The model under review builds one solid part; all positions refer to its coordinate system, in mm. Face numbers are marked on the shaded views. A direction names the side the tool comes from. Give positions to 0.01 mm unless a question says otherwise; leave off trailing zeros. Loops run counter-clockwise (first coordinate to the right, second up) from the corner with the lowest first, then second, coordinate; pieces in that order, holes last. Notation, with made-up numbers: (1.5, 76) - (18.5, 76) arc R34 cw to (18.5, 106) - close; hole circle Ø3 at (65.5, 54). An arc over 180 degrees is marked (long way). Return JSON: item names as keys, results as strings. Group by question number.
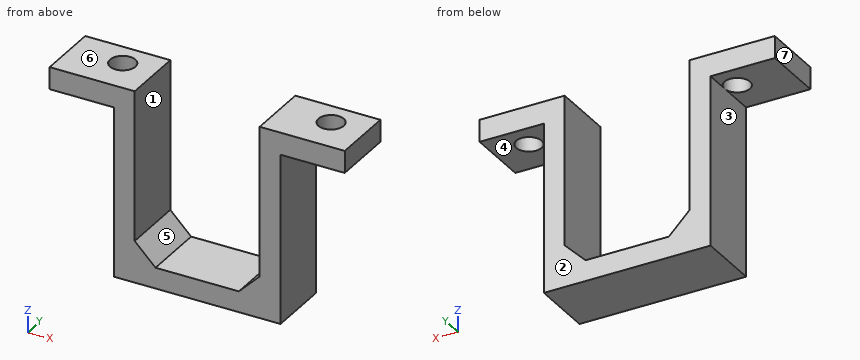
from build123d import *

# Parameters (mm, degrees)
BOSS_EXTRUDE1_DEPTH = 15
SKETCH3_R           = 3.05
CUT_EXTRUDE1_DEPTH  = 15


with BuildPart() as part:
    # Sketch2 → Boss-Extrude1 (new body)
    with BuildSketch(Plane(origin=(0, 0, 0), x_dir=(1, 0, 0), z_dir=(0, 1, 0))):
        Polygon((-13.5, 0), (6.5, 0), (11.5, -5), (11.5, -41), (31.917309801, -41), (31.917309801, -35.69895288), (16.5, -35.69895288), (16.5, 5), (-23.5, 5), (-23.5, -35.69895288), (-38.917309801, -35.69895288), (-38.917309801, -41), (-18.5, -41), (-18.5, -5), align=None)
    extrude(amount=BOSS_EXTRUDE1_DEPTH)

    # Sketch3 → Cut-Extrude1 (cut)
    with BuildSketch(Plane(origin=(0, 0, 35.69895288), x_dir=(-1, 0, 0), z_dir=(0, 0, -1))):
        with Locations((26.5, 9)):
            Circle(SKETCH3_R)
        with Locations((-23.5, 9)):
            Circle(SKETCH3_R)
    extrude(amount=-CUT_EXTRUDE1_DEPTH, mode=Mode.SUBTRACT)


solid = part.part
Item 1: Take a section at B-B (z = 29). State the section outline as (x, y) points, then the cut area to 3 significant figures.
Item 2: Take a section at D-D (x = 23.5). State the section outline as (y, z) points, then the cut area to 3 significant figures.
Item 3: Take a section at A-A (z = 37). State the section outline as (x, y) points.
Item 4: For L1, parallel to X at y = 9, z = 20.5; L2, parallel to X at y = 8, z = 37; L3, parallel to Z at x = -31.5, y = 12.75, list the stretches that pass through material, from the lowest coordinate up. Write a range as from..to.
Item 5: Take a section at C-C (y = 10.5). State the section outline as (x, z) points.
Item 6: Tool access review of the marked faces 1, 2, 3 and 4: name each direction out of +Z, -Z, +X, -X, +Y, -Y from which nothing blocks a thin tool from reaching the whole face with its end or side.
Item 7: For P1, Ø4.5, axis at y = 7.5, z = 30.5, coming from the +X side; P2, Ø3, axis at y = 6, z = 6, coming from the -X side; P3, Ø7, axis at x = 23.5, y = 9, coming from the -Z side, all flat-tipped, find the tip position at first contact; note any pin that passes through.
Item 8: Mouldability with a two-part tool opening along X and no side actions: class the marked faces 5, 6 and 7 as +X half, -X half, draft (parallel to the pull), parting line (faces both ways), or undercut.
Check sheet entries:
{
 "1": {"outline": "(-23.5, 0) - (-18.5, 0) - (-18.5, 15) - (-23.5, 15) - close; (11.5, 0) - (16.5, 0) - (16.5, 15) - (11.5, 15) - close", "area": "150 mm^2"},
 "2": {"outline": "(0, 35.7) - (5.95, 35.7) - (5.95, 41) - (0, 41) - close; (12.05, 35.7) - (15, 35.7) - (15, 41) - (12.05, 41) - close", "area": "47.2 mm^2"},
 "3": {"outline": "(-38.92, 0) - (-18.5, 0) - (-18.5, 15) - (-38.92, 15) - close; (11.5, 0) - (31.92, 0) - (31.92, 15) - (11.5, 15) - close; hole circle Ø6.1 at (-26.5, 9); hole circle Ø6.1 at (23.5, 9)"},
 "4": {"L1": "x = -23.5..-18.5, 11.5..16.5", "L2": "x = -38.92..-29.38, -23.62..-18.5, 11.5..20.62, 26.38..31.92", "L3": "z = 35.7..41"},
 "5": {"outline": "(-38.92, 35.7) - (-29.16, 35.7) - (-29.16, 41) - (-38.92, 41) - close; (-23.84, 35.7) - (-23.5, 35.7) - (-23.5, -5) - (16.5, -5) - (16.5, 35.7) - (20.84, 35.7) - (20.84, 41) - (11.5, 41) - (11.5, 5) - (6.5, 0) - (-13.5, 0) - (-18.5, 5) - (-18.5, 41) - (-23.84, 41) - close; (26.16, 35.7) - (31.92, 35.7) - (31.92, 41) - (26.16, 41) - close"},
 "6": {"face 1": "+Z, +Y, -Y", "face 2": "+Z, -Z, +X, -X, +Y", "face 3": "-Z, -X, +Y, -Y", "face 4": "-Z, +X, +Y, -Y"},
 "7": {"P1": "stops at x = 16.5", "P2": "stops at x = -23.5", "P3": "stops at z = 35.7"},
 "8": {"face 5": "undercut", "face 6": "draft", "face 7": "-X half"}
}
